Check sheet for the drawn part. Datum: minimum x, y, z corner. Units: mm. Give positions to 0.01 mm unless a question says otherwise; leave off trailing zeros. Loops run counter-clockwise (first coordinate to the right, second up) from the corner with the lowest first, then second, coordinate; pieces in that order, holes last. Notation, with made-up numbers: (-4.5, 4) - (4.5, 4) arc R15 cw to (4.5, 21) - close; hole circle Ø3 at (13, 46.25). An arc over 180 degrees is marked (long way). Use a Markdown table: item, result. Add a question column.
1. Cross-section at A-A on x = 19. Enter the section's corners in (y, z), and give its area (3 significant figures).
2. Material ranges on L1, parallel to Y at x = 21.25, z = 3; L2, parallel to X at y = 45.5, z = 3.2; L3, parallel to Y at x = 57, z = 3.7, recorded low to high.
3. Cross-section at B-B on y = 14.5. Enter the section's corners in (x, z) (3 decimals), and give its area (3 significant figures).
4. Cross-section at C-C on z = 3. Count the separate pieces of the cut face and the enclosed holes in it, and give its area (3 significant figures).
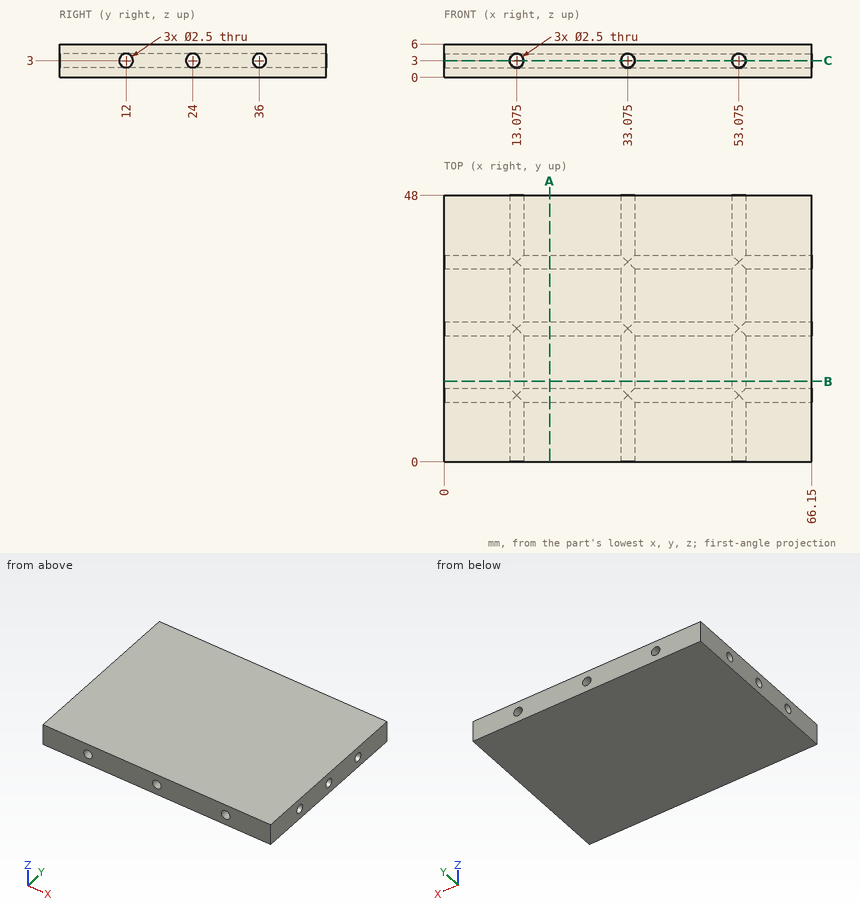
Values found:
| question | item | result |
|---|---|---|
| 1 | outline | (0, 0) - (48, 0) - (48, 6) - (0, 6) - close; hole circle Ø2.5 at (12, 3); hole circle Ø2.5 at (24, 3); hole circle Ø2.5 at (36, 3) |
| 1 | area | 273 mm2 |
| 2 | L1 | y = 0 to 10.75, 13.25 to 22.75, 25.25 to 34.75, 37.25 to 48 |
| 2 | L2 | x = 0 to 11.84, 14.31 to 31.84, 34.31 to 51.84, 54.31 to 66.15 |
| 2 | L3 | y = 0 to 10.96, 13.04 to 22.96, 25.04 to 34.96, 37.04 to 48 |
| 3 | outline | (0, 0) - (66.15, 0) - (66.15, 6) - (0, 6) - close; hole circle Ø2.5 at (13.075, 3); hole circle Ø2.5 at (33.075, 3); hole circle Ø2.5 at (53.075, 3) |
| 3 | area | 382 mm2 |
| 4 | separate pieces | 16 |
| 4 | enclosed holes | 0 |
| 4 | area | 2,380 mm2 |
